from build123d import *

# Parameters (mm, degrees)
F0_W     = 5
F0_H     = 2
F0_W_2   = 6
F1_DEPTH = 16
F2_DEPTH = 4
F3_DEPTH = 6
F4_DEPTH = 10


with BuildPart() as f1:
    # F0 (on Top) → F1 (new body)
    with BuildSketch(Plane.XY):
        with BuildLine():
            Line((-20, -2), (-14, -2))
            ThreePointArc((-14, -2), (-14.707107, -1.707107), (-15, -1))
            Line((-15, -1), (-15, 1))
            ThreePointArc((-15, 1), (-14.707107, 1.707107), (-14, 2))
            Line((-14, 2), (-20, 2))
            ThreePointArc((-20, 2), (-20.707107, 1.707107), (-21, 1))
            Line((-21, 1), (-21, -1))
            ThreePointArc((-21, -1), (-20.707107, -1.707107), (-20, -2))
        make_face()
        with BuildLine():
            Line((-14, -2), (14, -2))
            ThreePointArc((14, -2), (14.707107, -1.707107), (15, -1))
            Line((15, -1), (15, 1))
            ThreePointArc((15, 1), (14.707107, 1.707107), (14, 2))
            Line((14, 2), (-14, 2))
            ThreePointArc((-14, 2), (-14.707107, 1.707107), (-15, 1))
            Line((-15, 1), (-15, -1))
            ThreePointArc((-15, -1), (-14.707107, -1.707107), (-14, -2))
        make_face()
        Polygon((8, -1), (3, -1), (-3, -1), (-8, -1), (-8, 1), (-3, 1), (3, 1), (8, 1), align=None, mode=Mode.SUBTRACT)
        with Locations((-5.5, 0)):
            Rectangle(F0_W, F0_H)
        Rectangle(F0_W_2, F0_H)
        with Locations((5.5, 0)):
            Rectangle(F0_W, F0_H)
        with BuildLine():
            Line((14, -2), (20, -2))
            ThreePointArc((20, -2), (20.707107, -1.707107), (21, -1))
            Line((21, -1), (21, 1))
            ThreePointArc((21, 1), (20.707107, 1.707107), (20, 2))
            Line((20, 2), (14, 2))
            ThreePointArc((14, 2), (14.707107, 1.707107), (15, 1))
            Line((15, 1), (15, -1))
            ThreePointArc((15, -1), (14.707107, -1.707107), (14, -2))
        make_face()
    extrude(amount=-F1_DEPTH)

    # F0 (on Top) → F2 (join)
    with BuildSketch(Plane.XY):
        with BuildLine():
            Line((-14, -2), (14, -2))
            ThreePointArc((14, -2), (14.707107, -1.707107), (15, -1))
            Line((15, -1), (15, 1))
            ThreePointArc((15, 1), (14.707107, 1.707107), (14, 2))
            Line((14, 2), (-14, 2))
            ThreePointArc((-14, 2), (-14.707107, 1.707107), (-15, 1))
            Line((-15, 1), (-15, -1))
            ThreePointArc((-15, -1), (-14.707107, -1.707107), (-14, -2))
        make_face()
        Polygon((8, -1), (3, -1), (-3, -1), (-8, -1), (-8, 1), (-3, 1), (3, 1), (8, 1), align=None, mode=Mode.SUBTRACT)
    extrude(amount=F2_DEPTH)

    # F0 (on Top) → F3 (join)
    with BuildSketch(Plane.XY):
        with Locations((-5.5, 0)):
            Rectangle(F0_W, F0_H)
        with Locations((5.5, 0)):
            Rectangle(F0_W, F0_H)
    extrude(amount=F3_DEPTH)

    # F0 (on Top) → F4 (join)
    with BuildSketch(Plane.XY):
        Rectangle(F0_W_2, F0_H)
    extrude(amount=F4_DEPTH)


solid = f1.part
Here's how the part is built. I have some questions about the finished solid (model axes, mm). A direction names the side the tool comes from. Coordinates: 2 decimals unless noted, no trailing zeros. Order: outer loops, then holes, each group sorted by start corner. A loop starts at its lowest first (then second) coordinate and runs counter-clockwise, first axis right, second up.
Item 1: If we section it at D-D on x = -17: List the corners of the cut face in (y, z) for me.
Result sheet:
outline: (-2, -16) - (2, -16) - (2, 0) - (-2, 0) - close
Item 2: If we section it at A-A on y = -0.25: List the corners of the cut face in (x, z) for me.
Result sheet:
outline: (-21, -16) - (21, -16) - (21, 0) - (15, 0) - (15, 4) - (8, 4) - (8, 6) - (3, 6) - (3, 10) - (-3, 10) - (-3, 6) - (-8, 6) - (-8, 4) - (-15, 4) - (-15, 0) - (-21, 0) - close
Item 3: I need wall thicknesses on line 1 (Z direction, x = -16.5, y = 0.05); line 2 (X direction, y = 0.3, z = 6.5); line 3 (Z direction, x = 8.5, y = 1.3). Which ranges of each line are inside material? Lowest first, please.
Result sheet:
line 1: z = -16 to 0
line 2: x = -3 to 3
line 3: z = -16 to 4
Item 4: For faces 1 (the face through (5, 0, 6)), 2 (the face through (-14.715, -1.699, 1.972)), 3 (the face through (-14.699, 1.715, 1.972)), 4 (the face through (-3, 0, 8)), which set-ups out of +Z, -Z, +X, -X, +Y, -Y let a thin tool reach every point of the face, with its end or its side?
Result sheet:
face 1: +Z, +X, +Y, -Y
face 2: +Z, -X, -Y
face 3: +Z, -X, +Y
face 4: +Z, -X, +Y, -Y
Item 5: If we section it at B-B on z = 3.5: List the corners of the cut face in (x, y) for me.
Result sheet:
outline: (-15, -1) arc R1 ccw to (-14, -2) - (14, -2) arc R1 ccw to (15, -1) - (15, 1) arc R1 ccw to (14, 2) - (-14, 2) arc R1 ccw to (-15, 1) - close
Item 6: For P1, Ø2, axis at x = 5.5, y = 0.5, coming from the +Z side; P2, Ø2, axis at y = 0, z = 2.5, coming from the -X side; P3, Ø2, axis at y = -0.5, z = 5.5, coming from the -X side, each with a flat end and sliding along its axis, tell me the tip position at first contact or that it passes through.
Result sheet:
P1: stops at z = 6
P2: stops at x = -15
P3: stops at x = -8
Item 7: If we section it at C-C on x = 0: List the corners of the cut face in (y, z) for me, plus the area to 3 significant figures.
Result sheet:
outline: (-2, -16) - (2, -16) - (2, 4) - (1, 4) - (1, 10) - (-1, 10) - (-1, 4) - (-2, 4) - close
area: 92.0 mm2
